```python
from build123d import *

# Parameters (mm, degrees)
SKETCH_2_R          = 22.5
SKETCH_2_R_2        = 2.0999999999999956
SKETCH_2_R_3        = 2.1
SKETCH_2_R_4        = 2.0999999999999974
SKETCH_2_R_5        = 6
EXTRUDE_1_DEPTH     = 1.5
EXTRUDE_START       = 10
SKETCH_4_R          = 22.500000000000004
SKETCH_4_R_2        = 21
EXTRUDE_2_DEPTH     = 10
EXTRUDE_3_DEPTH     = 10
SKETCH_6_R          = 8
SKETCH_6_R_2        = 7
EXTRUDE_4_DEPTH     = 4
EXTRUDE_5_DEPTH     = 2
CHAMFER_1_SIZE      = 0.5
EXTRUDE_START_2     = 21.5
SKETCH_9_R          = 3
EXTRUDE_6_DEPTH     = 5
EXTRUDE_6_TAPER     = 10.000000000000021
SKETCH_10_R         = 1
CUT_EXTRUDE_1_DEPTH = 5


with BuildPart() as part:
    # 草图2 → 凸台-拉伸1 (new body)
    with BuildSketch(Plane(origin=(0, 0, 0), x_dir=(1, 0, 0), z_dir=(0, 1, 0))):
        with Locations(Location((0, 0, 0), (0, 0, 270))):
            Circle(SKETCH_2_R)
        with Locations(Location((14, 0, 0), (0, 0, 270))):
            Circle(SKETCH_2_R_2, mode=Mode.SUBTRACT)
        with Locations(Location((0, 14, 0), (0, 0, 270))):
            Circle(SKETCH_2_R_3, mode=Mode.SUBTRACT)
        with Locations(Location((0, -14, 0), (0, 0, 90))):
            Circle(SKETCH_2_R_3, mode=Mode.SUBTRACT)
        with Locations(Location((-13.999999999999993, -3.43e-15, 0), (0, 0, 90))):
            Circle(SKETCH_2_R_4, mode=Mode.SUBTRACT)
        with Locations(Location((0, 0, 0), (0, 0, 270))):
            Circle(SKETCH_2_R_5, mode=Mode.SUBTRACT)
    extrude(amount=EXTRUDE_1_DEPTH)

    # 草图4 → 凸台-拉伸2 (add)
    with BuildSketch(Plane.XZ.offset(EXTRUDE_START)):
        with Locations(Location((0, 0, 0), (0, 0, 270))):
            Circle(SKETCH_4_R)
        with Locations(Location((0, 0, 0), (0, 0, 270))):
            Circle(SKETCH_4_R_2, mode=Mode.SUBTRACT)
    extrude(amount=-EXTRUDE_2_DEPTH)

    # 草图5 → 凸台-拉伸3 (add)
    with BuildSketch(Plane(origin=(0, 1.5, 0), x_dir=(1, 0, 0), z_dir=(0, 1, 0))):
        Polygon((26.8, 0.9), (26.8, -0.9), (21, -0.9000000000000008), (21, 0.9000000000000008), align=None)
        Polygon((12.620577136594008, -23.659480821422953), (9.720577136594008, -18.63653347947321), (11.279422863405998, -17.736533479473213), (14.179422863405998, -22.759480821422954), align=None)
        Polygon((-14.179422863405991, -22.759480821422965), (-11.279422863405994, -17.736533479473213), (-9.720577136594002, -18.636533479473215), (-12.620577136594001, -23.65948082142296), align=None)
        Polygon((-26.8, 0.8999999999999966), (-21, 0.8999999999999982), (-21, -0.9000000000000035), (-26.8, -0.9000000000000032), align=None)
        Polygon((-12.620577136594019, 23.65948082142295), (-9.720577136594015, 18.63653347947321), (-11.279422863406003, 17.73653347947321), (-14.179422863406007, 22.75948082142295), align=None)
        Polygon((14.179422863405977, 22.75948082142297), (11.279422863405983, 17.736533479473216), (9.72057713659399, 18.63653347947322), (12.620577136593988, 23.659480821422964), align=None)
    extrude(amount=-EXTRUDE_3_DEPTH)

    # 草图6 → 凸台-拉伸4 (add)
    # profile 1 of 5: a face of its own
    with BuildSketch(Plane(origin=(0, 1.5, 0), x_dir=(1, 0, 0), z_dir=(0, 1, 0))):
        with Locations(Location((0, 0, 0), (0, 0, 270))):
            Circle(SKETCH_6_R)
        with Locations(Location((0, 0, 0), (0, 0, 270))):
            Circle(SKETCH_6_R_2, mode=Mode.SUBTRACT)
    # profile 2 of 5: a face of its own
    with BuildSketch(Plane(origin=(0, 1.5, 0), x_dir=(1, 0, 0), z_dir=(0, 1, 0))):
        with BuildLine():
            ThreePointArc((16.42857142857143, 4.370588154508102), (12.02081528017131, 12.020815280171309), (4.370588154508102, 16.42857142857143))
            ThreePointArc((4.370588154508102, 16.42857142857143), (4.74213736554837, 15.584971042722852), (4.952508833914383, 14.6875))
            ThreePointArc((4.952508833914383, 14.6875), (10.960155108391488, 10.960155108391486), (14.687500000000002, 4.952508833914381))
            ThreePointArc((14.687500000000002, 4.952508833914381), (15.584971042722852, 4.742137365548372), (16.42857142857143, 4.370588154508102))
        make_face()
    # profile 3 of 5: a face of its own
    with BuildSketch(Plane(origin=(0, 1.5, 0), x_dir=(1, 0, 0), z_dir=(0, 1, 0))):
        with BuildLine():
            ThreePointArc((4.370588154508102, -16.42857142857143), (4.742137365548372, -15.584971042722852), (4.952508833914385, -14.6875))
            ThreePointArc((4.952508833914385, -14.6875), (10.960155108391488, -10.960155108391486), (14.687500000000002, -4.952508833914381))
            ThreePointArc((14.687500000000002, -4.952508833914381), (15.584971042722852, -4.742137365548368), (16.42857142857143, -4.370588154508102))
            ThreePointArc((16.42857142857143, -4.370588154508102), (12.02081528017131, -12.020815280171309), (4.370588154508102, -16.42857142857143))
        make_face()
    # profile 4 of 5: a face of its own
    with BuildSketch(Plane(origin=(0, 1.5, 0), x_dir=(1, 0, 0), z_dir=(0, 1, 0))):
        with BuildLine():
            ThreePointArc((-14.687500000000002, 4.952508833914374), (-15.584971042722852, 4.742137365548359), (-16.42857142857143, 4.370588154508093))
            ThreePointArc((-16.42857142857143, 4.370588154508093), (-12.020815280171314, 12.020815280171306), (-4.370588154508102, 16.42857142857143))
            ThreePointArc((-4.370588154508102, 16.42857142857143), (-4.742137365548372, 15.584971042722854), (-4.952508833914383, 14.6875))
            ThreePointArc((-4.952508833914383, 14.6875), (-10.960155108391486, 10.960155108391488), (-14.687500000000002, 4.952508833914374))
        make_face()
    # profile 5 of 5: a face of its own
    with BuildSketch(Plane(origin=(0, 1.5, 0), x_dir=(1, 0, 0), z_dir=(0, 1, 0))):
        with BuildLine():
            ThreePointArc((-4.952508833914385, -14.6875), (-4.742137365548372, -15.584971042722854), (-4.370588154508102, -16.42857142857143))
            ThreePointArc((-4.370588154508102, -16.42857142857143), (-12.020815280171309, -12.02081528017131), (-16.42857142857143, -4.370588154508101))
            ThreePointArc((-16.42857142857143, -4.370588154508101), (-15.584971042722854, -4.742137365548372), (-14.687500000000002, -4.952508833914382))
            ThreePointArc((-14.687500000000002, -4.952508833914382), (-10.960155108391486, -10.960155108391488), (-4.952508833914385, -14.6875))
        make_face()
    extrude(amount=EXTRUDE_4_DEPTH)

    # 草图7 → 凸台-拉伸5 (add)
    with BuildSketch(Plane(origin=(0, 1.5, 0), x_dir=(1, 0, 0), z_dir=(0, 1, 0))):
        with BuildLine():
            Line((14.687500000000002, -4.952508833914384), (7.580645161290323, -2.5561335916977446))
            ThreePointArc((7.580645161290323, -2.5561335916977446), (5.6568542494923815, -5.656854249492379), (2.5561335916977472, -7.580645161290323))
            Line((2.5561335916977472, -7.580645161290323), (4.952508833914385, -14.6875))
            ThreePointArc((4.952508833914385, -14.6875), (10.960155108391488, -10.960155108391486), (14.687500000000002, -4.952508833914384))
        make_face()
        with BuildLine():
            Line((-4.952508833914393, -14.6875), (-2.5561335916977583, -7.580645161290323))
            ThreePointArc((-2.5561335916977583, -7.580645161290323), (-5.656854249492388, -5.656854249492378), (-7.580645161290336, -2.5561335916977517))
            Line((-7.580645161290336, -2.5561335916977517), (-14.687500000000014, -4.952508833914387))
            ThreePointArc((-14.687500000000014, -4.952508833914387), (-10.960155108391493, -10.960155108391485), (-4.952508833914393, -14.6875))
        make_face()
        with BuildLine():
            Line((-14.687500000000014, 4.952508833914387), (-7.580645161290336, 2.5561335916977517))
            ThreePointArc((-7.580645161290336, 2.5561335916977517), (-5.656854249492388, 5.656854249492378), (-2.5561335916977583, 7.580645161290323))
            Line((-2.5561335916977583, 7.580645161290323), (-4.952508833914393, 14.6875))
            ThreePointArc((-4.952508833914393, 14.6875), (-10.960155108391493, 10.960155108391485), (-14.687500000000014, 4.952508833914387))
        make_face()
        with BuildLine():
            Line((4.952508833914385, 14.6875), (2.5561335916977472, 7.580645161290323))
            ThreePointArc((2.5561335916977472, 7.580645161290323), (5.6568542494923815, 5.656854249492379), (7.580645161290323, 2.5561335916977446))
            Line((7.580645161290323, 2.5561335916977446), (14.687500000000002, 4.952508833914381))
            ThreePointArc((14.687500000000002, 4.952508833914381), (10.960155108391488, 10.960155108391486), (4.952508833914385, 14.6875))
        make_face()
    extrude(amount=EXTRUDE_5_DEPTH)

    # 倒角1
    chamfer_1_edges = [part.edges().sort_by_distance(p)[0] for p in [
        (-26.8, -3.5, -0.8999999999999966),
        (-26.8, -8.5, 3.33e-15),
        (-26.8, -3.5, 0.9000000000000032),
        (-26.8, 1.5, 3.33e-15),
        (-12.620577136594019, -3.5, -23.65948082142295),
        (-13.400000000000013, -8.5, -23.20948082142295),
        (-14.179422863406007, -3.5, -22.75948082142295),
        (-13.400000000000013, 1.5, -23.20948082142295),
        (14.179422863405977, -3.5, -22.75948082142297),
        (13.399999999999983, -8.5, -23.209480821422964),
        (12.620577136593988, -3.5, -23.659480821422964),
        (13.399999999999983, 1.5, -23.209480821422964),
        (26.8, -3.5, 0.9),
        (26.8, -8.5, 0),
        (26.8, -3.5, -0.9),
        (26.8, 1.5, 0),
        (12.620577136594008, -3.5, 23.659480821422953),
        (13.400000000000002, -8.5, 23.209480821422954),
        (14.179422863405998, -3.5, 22.759480821422954),
        (13.400000000000002, 1.5, 23.209480821422954),
        (-14.179422863405991, -3.5, 22.759480821422965),
        (-13.399999999999995, -8.5, 23.209480821422964),
        (-12.620577136594001, -3.5, 23.65948082142296),
        (-13.399999999999995, 1.5, 23.209480821422964),
    ]]
    chamfer(chamfer_1_edges, length=CHAMFER_1_SIZE)

    # 草图9 → 凸台-拉伸6 (add)
    with BuildSketch(Plane.XY.offset(EXTRUDE_START_2)):
        with Locations((8.6e-16, -7)):
            Circle(SKETCH_9_R)
    extrude(amount=EXTRUDE_6_DEPTH, taper=EXTRUDE_6_TAPER)

    # 草图10 → 切除-拉伸1 (cut)
    with BuildSketch(Plane.XY.offset(26.5)):
        with Locations((8.6e-16, -7)):
            Circle(SKETCH_10_R)
    extrude(amount=-CUT_EXTRUDE_1_DEPTH, mode=Mode.SUBTRACT)


solid = part.part
```
Could you check a few things on this model? Use its own coordinates, in mm. A direction names the side the tool comes from. Coordinates: 2 decimals unless noted, no trailing zeros. Write each loop counter-clockwise with the first axis right and the second up, starting at its lowest first coordinate (ties: lowest second). Pieces come first, ordered by that corner, then holes. Notation, with made-up numbers: (-40, 36.5) - (-20, 36.5) arc R30 ccw to (-20, 70.5) - close; hole circle Ø11 at (52, 20). An arc over 180 degrees is marked (long way). Use a Markdown table: item, result.
Q1. Imagine slicing it at B-B (x = -9.5). List the corners of the cut face in (y, z) for me.
Geometry check:
| item | result |
|---|---|
| outline | (-10, -20.4) - (1.5, -20.4) - (1.5, -14.1) - (5.5, -14.1) - (5.5, -12.25) - (3.5, -12.25) - (3.5, -3.2) - (1.5, -3.2) - (1.5, 3.2) - (3.5, 3.2) - (3.5, 12.25) - (5.5, 12.25) - (5.5, 14.1) - (1.5, 14.1) - (1.5, 20.4) - (-10, 20.4) - (-10, 18.73) - (0, 18.73) - (0, -18.73) - (-10, -18.73) - close |
Q2. I'm going to push flat-ended pins straight in: pin 1 Ø6.5 at (x, z) = (-14, 0) entering from +Y; pin 2 Ø1.5 at (x, y) = (9.5, -1) entering from +Z; pin 3 Ø1 at (x, z) = (11.5, 22) entering from -Y; pin 4 Ø8.5 at (x, z) = (0, 0) entering from -Y. Where does each tip first touch, or does it pass through?
Geometry check:
| item | result |
|---|---|
| pin 1 | stops at y = 1.5 |
| pin 2 | stops at z = 20.73 |
| pin 3 | stops at y = -8.5 |
| pin 4 | passes through |
Q3. Please list where these lines run through material, in increasing order: L1, parallel to X at y = 0.75, z = 0; L2, parallel to X at y = -5.25, z = 0; L3, parallel to Y at x = -8, z = 18.
Geometry check:
| item | result |
|---|---|
| L1 | x = -26.8 to -16.1, -11.9 to -6, 6 to 11.9, 16.1 to 26.8 |
| L2 | x = -26.8 to -21, 21 to 26.8 |
| L3 | y = 0 to 1.5 |
Q4. Imagine slicing it at A-A (z = 14). List the corners of the cut face in (x, y) for me.
Geometry check:
| item | result |
|---|---|
| outline | (-17.61, -10) - (-15.65, -10) - (-15.65, 0) - (-2.1, 0) - (-2.1, 1.5) - (-4.72, 1.5) - (-4.72, 3.5) - (-6.65, 3.5) - (-6.65, 5.5) - (-9.64, 5.5) - (-9.64, 1.5) - (-17.61, 1.5) - close; (2.1, 0) - (15.65, 0) - (15.65, -10) - (17.61, -10) - (17.61, 1.5) - (9.64, 1.5) - (9.64, 5.5) - (6.65, 5.5) - (6.65, 3.5) - (4.72, 3.5) - (4.72, 1.5) - (2.1, 1.5) - close |
Q5. Which directions (+Z, -Z, +X, -X, +Y, -Y) give clear straight access to the entire face, cutting with the end or side of a thin tool? Please do faces 1 (the cylindrical face through (12.11, 3.47, -11.93)), 2 (the flat face through (-24, -3, -0.9)), 3 (the flat face through (24, -8.5, 0)), 4 (the cylindrical face through (4.738, 3.472, -15.597)), 5 (the cylindrical face through (-12.11, 3.47, -11.93)).
Geometry check:
| item | result |
|---|---|
| face 1 | -Z, +X, +Y |
| face 2 | -Z, -X, +Y, -Y |
| face 3 | +Z, -Z, +X, -Y |
| face 4 | +Y |
| face 5 | -Z, -X, +Y |
Q6. Imagine slicing it at C-C (z = -11). List the corners of the cut face in (x, y) for me.
Geometry check:
| item | result |
|---|---|
| outline | (-19.63, -10) - (-17.89, -10) - (-17.89, 0) - (17.89, 0) - (17.89, -10) - (19.63, -10) - (19.63, 1.5) - (12.96, 1.5) - (12.96, 5.5) - (10.92, 5.5) - (10.92, 3.5) - (3.71, 3.5) - (3.71, 1.5) - (-3.71, 1.5) - (-3.71, 3.5) - (-10.92, 3.5) - (-10.92, 5.5) - (-12.96, 5.5) - (-12.96, 1.5) - (-19.63, 1.5) - close |
Q7. Thinking about a two-plate mould opening in Y: for faces 6 (the flat face through (0, -7, 21.5)), 7 (the flat face through (1, -6, 26.5)), 8 (the flat face through (-6, 1.5, -2)), which applies, +Y half, -Y half, draft (parallel to the pull), parting line (faces both ways), or undercut?
Geometry check:
| item | result |
|---|---|
| face 6 | undercut |
| face 7 | draft |
| face 8 | +Y half |
